Can you work these out from the model? Positions are in its coordinate system, mm. Face numbers are marked on the shaded views. A direction names the side the tool comes from. Round coordinates to 2 decimals unless told otherwise and drop trailing zeros. Write each loop counter-clockwise with the first axis right and the second up, starting at its lowest first coordinate (ties: lowest second). Pieces come first, ordered by that corner, then holes. Notation, with made-up numbers: M 24,52.5 L 69,52.5 A12 cw 69,58.5 Z; hole C 67,81 d4. An arc over 180 degrees is marked long. Use one line per item in the form item = value. Start each with the question number.
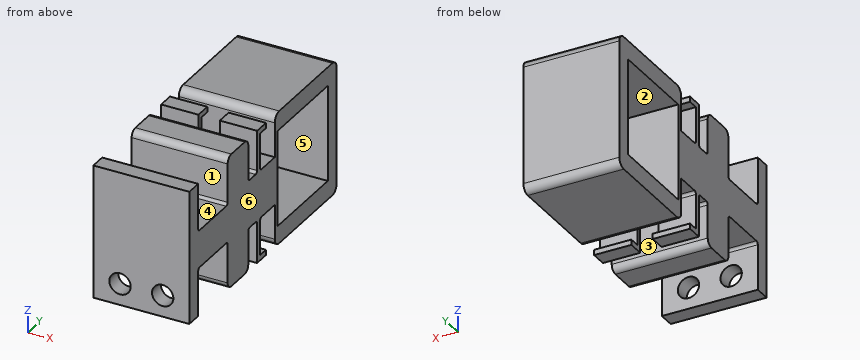
Autodesk Fusion 360 part; units mm, degrees
sketch "Sketch1" plane through (0, 0, 0) normal (1, 0, 0) x (0, 0, -1)
  line L0 (0, 0) -> (-18, 0)
  line L1 (-18, 0) -> (-18, 17)
  line L2 (-18, 17) -> (0, 17)
  line L3 (0, 17) -> (0, 0)
  line L4 (-21.5, 20) -> (3.5, 20)
  line L5 (3.5, 20) -> (3.5, -30)
  line L6 (3.5, -30) -> (-21.5, -30)
  line L7 (-21.5, -30) -> (-21.5, 20)
  dimension "d1" = 18
  dimension "d2" = 17
  dimension "d3" = 25
  dimension "d4" = 50
  dimension "d66" = 3.5
extrude "Extrude1" add sketch "Sketch1" against normal blind 18
fillet "Fillet1" radius 1.5 2 edges at (-9, 20, -3.5) (-9, 20, 21.5)
sketch "Sketch2" plane through (0, 0, 0) normal (1, 0, 0) x (0, 0, -1)
  line L0 (-18, 17) -> (0, 17)
  line L1 (0, 17) -> (0, 0)
  line L2 (0, 0) -> (-18, 0)
  line L3 (-18, 0) -> (-18, 17)
  arc A0 (-20, 20) -> (-21.5, 18.5) centre (-20, 18.5) ccw
  line L4 (-21.5, 18.5) -> (-21.5, -30)
  line L5 (-21.5, -30) -> (3.5, -30)
  line L6 (3.5, -30) -> (3.5, 18.5)
  arc A1 (3.5, 18.5) -> (2, 20) centre (2, 18.5) ccw
  line L7 (2, 20) -> (-20, 20)
  line L8 (-21.5, -3.9907) -> (-20.5, -3.9907)
  line L9 (-20.5, -3.9907) -> (-20.5, -6)
  line L10 (-20.5, -6) -> (-13.5, -6)
  line L11 (-13.5, -6) -> (-13.5, -0.9907)
  line L12 (-13.5, -0.9907) -> (-21.5, -0.9907)
  line L13 (3.5, -1) -> (-4.5, -1)
  line L14 (-4.5, -1) -> (-4.5, -6)
  line L15 (-4.5, -6) -> (2.5, -6)
  line L16 (2.5, -6) -> (2.5, -4)
  line L17 (2.5, -4) -> (3.5, -4)
  dimension "d9" = 7
  dimension "d10" = 8
  dimension "d12" = 5.0093
  dimension "d13" = 1
  dimension "d14" = 3
  dimension "d15" = 3
  dimension "d16" = 5
  dimension "d17" = 1
extrude "Extrude2" cut sketch "Sketch2" against normal blind 43 contours L4 L8 L9 L10 L11 L12 | L6 L13 L14 L15 L16 L17
sketch "Sketch3" plane through (0, 0, 21.5) normal (0, 0, 1) x (1, 0, 0)
  line L0 (0, -3.9907) -> (-18, -3.9907)
  line L1 (-18, -3.9907) -> (-18, -30)
  line L2 (-18, -30) -> (0, -30)
  line L3 (0, -30) -> (0, -3.9907)
  line L4 (0, -3.9907) -> (-7, -3.9907)
  line L5 (-7, -3.9907) -> (-7, -5.9907)
  line L6 (-7, -5.9907) -> (0, -5.9907)
  line L7 (0, -5.9907) -> (0, -3.9907)
  line L8 (-18, -3.9907) -> (-11, -3.9907)
  line L9 (-11, -3.9907) -> (-11, -5.9907)
  line L10 (-11, -5.9907) -> (-18, -5.9907)
  line L11 (-18, -5.9907) -> (-18, -3.9907)
  line L12 (-11, -3.9907) -> (-7, -3.9907)
  line L13 (-7, -3.9907) -> (-7, -5.9907)
  line L14 (-7, -5.9907) -> (-11, -5.9907)
  line L15 (-11, -5.9907) -> (-11, -3.9907)
  dimension "d21" = 7
  dimension "d22" = 2
  dimension "d23" = 7
  dimension "d24" = 2
extrude "Extrude3" cut sketch "Sketch3" against normal blind 8 contours L0 L5 L9 L12 L13 L14 L15
sketch "Sketch4" plane through (0, 0, -3.5) normal (0, 0, -1) x (-1, 0, 0)
  line L0 (18, -4) -> (0, -4)
  line L1 (0, -4) -> (0, -30)
  line L2 (0, -30) -> (18, -30)
  line L3 (18, -30) -> (18, -4)
  line L4 (0, -4) -> (7, -4)
  line L5 (7, -4) -> (7, -6)
  line L6 (7, -6) -> (0, -6)
  line L7 (0, -6) -> (0, -4)
  line L8 (18, -4) -> (11, -4)
  line L9 (11, -4) -> (11, -6)
  line L10 (11, -6) -> (18, -6)
  line L11 (18, -6) -> (18, -4)
  line L12 (7, -4) -> (11, -4)
  line L13 (11, -4) -> (11, -6)
  line L14 (11, -6) -> (7, -6)
  line L15 (7, -6) -> (7, -4)
  dimension "d27" = 7
  dimension "d28" = 2
  dimension "d29" = 7
  dimension "d30" = 2
extrude "Extrude4" cut sketch "Sketch4" against normal blind 8 contours L0 L5 L9 L12 L13 L14 L15
sketch "Sketch5" plane through (0, 0, -3.5) normal (0, 0, -1) x (-1, 0, 0)
  line L0 (7, -6) -> (7, -4)
  line L1 (7, -4) -> (0, -4)
  line L2 (0, -4) -> (0, -30)
  line L3 (0, -30) -> (18, -30)
  line L4 (18, -30) -> (18, -4)
  line L5 (18, -4) -> (11, -4)
  line L6 (11, -4) -> (11, -6)
  line L7 (11, -6) -> (7, -6)
  line L8 (7, -4) -> (11, -4)
  line L9 (11, -4) -> (11, -10)
  line L10 (11, -10) -> (7, -10)
  line L11 (7, -10) -> (7, -4)
  line L12 (11, -10) -> (18, -10)
  line L13 (18, -10) -> (18, -7)
  line L14 (18, -7) -> (11, -7)
  line L15 (11, -7) -> (11, -10)
  line L16 (7, -10) -> (0, -10)
  line L17 (0, -10) -> (0, -7)
  line L18 (0, -7) -> (7, -7)
  line L19 (7, -7) -> (7, -10)
  dimension "d33" = 3
extrude "Extrude5" cut sketch "Sketch5" against normal blind 8 contours L0 L6 L7 L8 L9 L11 | L7 L9 L10 L11 L15 L19 | L2 L11 L16 L17 L18 L19 | L4 L9 L12 L13 L14 L15
sketch "Sketch6" plane through (0, 0, 21.5) normal (0, 0, 1) x (1, 0, 0)
  line L0 (-11, -5.9907) -> (-11, -3.9907)
  line L1 (-11, -3.9907) -> (-18, -3.9907)
  line L2 (-18, -3.9907) -> (-18, -30)
  line L3 (-18, -30) -> (0, -30)
  line L4 (0, -30) -> (0, -3.9907)
  line L5 (0, -3.9907) -> (-7, -3.9907)
  line L6 (-7, -3.9907) -> (-7, -5.9907)
  line L7 (-7, -5.9907) -> (-11, -5.9907)
  line L8 (-11, -5.9907) -> (-7, -5.9907)
  line L9 (-7, -5.9907) -> (-7, -9.9907)
  line L10 (-7, -9.9907) -> (-11, -9.9907)
  line L11 (-11, -9.9907) -> (-11, -5.9907)
  line L12 (-7, -9.9907) -> (0, -9.9907)
  line L13 (0, -9.9907) -> (0, -6.9907)
  line L14 (0, -6.9907) -> (-7, -6.9907)
  line L15 (-7, -6.9907) -> (-7, -9.9907)
  line L16 (-11, -9.9907) -> (-18, -9.9907)
  line L17 (-18, -9.9907) -> (-18, -6.9907)
  line L18 (-18, -6.9907) -> (-11, -6.9907)
  line L19 (-11, -6.9907) -> (-11, -9.9907)
  dimension "d36" = 4
  dimension "d37" = 3
  dimension "d38" = 3
  dimension "d39" = 7
extrude "Extrude6" cut sketch "Sketch6" against normal blind 8 contours L7 L8 L9 L10 L11 L15 L19 | L2 L11 L16 L17 L18 L19 | L4 L9 L12 L13 L14 L15
sketch "Sketch7" plane through (0, -30, 0) normal (0, -1, 0) x (1, 0, 0)
  line L0 (0, -3.5) -> (0, 21.5)
  line L1 (0, 21.5) -> (-18, 21.5)
  line L2 (-18, 21.5) -> (-18, -3.5)
  line L3 (-18, -3.5) -> (0, -3.5)
sketch "Sketch8" plane through (0, 0, 0) normal (1, 0, 0) x (0, 0, -1)
  line L0 (-13.5, -9.9907) -> (-21.5, -9.9907)
  line L1 (-21.5, -9.9907) -> (-21.5, -30)
  line L2 (-21.5, -30) -> (3.5, -30)
  line L3 (3.5, -30) -> (3.5, -10)
  line L4 (3.5, -10) -> (-4.5, -10)
  line L5 (-4.5, -10) -> (-4.5, -7)
  line L6 (-4.5, -7) -> (3.5, -7)
  line L7 (3.5, -7) -> (3.5, -4)
  line L8 (3.5, -4) -> (2.5, -4)
  line L9 (2.5, -4) -> (2.5, -6)
  line L10 (2.5, -6) -> (-4.5, -6)
  line L11 (-4.5, -6) -> (-4.5, -1)
  line L12 (-4.5, -1) -> (3.5, -1)
  line L13 (3.5, -1) -> (3.5, 18.5)
  arc A0 (3.5, 18.5) -> (2, 20) centre (2, 18.5) ccw
  line L14 (2, 20) -> (-20, 20)
  arc A1 (-20, 20) -> (-21.5, 18.5) centre (-20, 18.5) ccw
  line L15 (-21.5, 18.5) -> (-21.5, -0.9907)
  line L16 (-21.5, -0.9907) -> (-13.5, -0.9907)
  line L17 (-13.5, -0.9907) -> (-13.5, -6)
  line L18 (-13.5, -6) -> (-20.5, -6)
  line L19 (-20.5, -6) -> (-20.5, -3.9907)
  line L20 (-20.5, -3.9907) -> (-21.5, -3.9907)
  line L21 (-21.5, -3.9907) -> (-21.5, -6.9907)
  line L22 (-21.5, -6.9907) -> (-13.5, -6.9907)
  line L23 (-13.5, -6.9907) -> (-13.5, -9.9907)
  line L24 (-18, 17) -> (0, 17)
  line L25 (0, 17) -> (0, 0)
  line L26 (0, 0) -> (-18, 0)
  line L27 (-18, 0) -> (-18, 17)
  line L28 (-21.5, -30) -> (3.5, -30)
  line L29 (3.5, -30) -> (3.5, -27)
  line L30 (3.5, -27) -> (-21.5, -27)
  line L31 (-21.5, -27) -> (-21.5, -30)
  line L32 (-21.5, -27) -> (-12.5, -27)
  line L33 (-12.5, -27) -> (-12.5, -23)
  line L34 (-12.5, -23) -> (-21.5, -23)
  line L35 (-21.5, -23) -> (-21.5, -27)
  line L36 (3.5, -27) -> (-5.5, -27)
  line L37 (-5.5, -27) -> (-5.5, -23)
  line L38 (-5.5, -23) -> (3.5, -23)
  line L39 (3.5, -23) -> (3.5, -27)
  dimension "d42" = 3
extrude "Extrude7" cut sketch "Sketch8" against normal blind 32 contours L1 L30 L32 L33 L34 L35 | L3 L30 L36 L37 L38 L39
fillet "Fillet2" radius 0.5 8 edges at (-14.5, -6, 13.5) (-3.5, -6, 13.5) (-3.5, -6.9907, 13.5) (-14.5, -6.9907, 13.5) (-3.5, -7, 4.5) (-3.5, -6, 4.5) (-14.5, -6, 4.5) (-14.5, -7, 4.5)
sketch "Sketch9" plane through (0, -30, 0) normal (0, -1, 0) x (1, 0, 0)
  line L0 (0, 20) -> (-18, 20)
  line L1 (-18, 20) -> (-18, -5)
  line L2 (-18, -5) -> (0, -5)
  line L3 (0, -5) -> (0, 20)
  line L4 (0, 20) -> (0, 7.5)
  line L5 (0, 7.5) -> (-18, 7.5)
  line L6 (-18, 7.5) -> (-13, 7.5)
  circle A0 centre (-13, 0.5) radius 2
  line L7 (-9, -5) -> (-9, 20)
  circle A1 centre (-5, 0.5) radius 2
  dimension "d50" = 4
  dimension "d63" = 4
  dimension "d64" = 4
  dimension "d65" = 4
extrude "Extrude8" cut sketch "Sketch9" against normal blind 5 contours A0 | A1
extrude "Extrude9" cut 2 faces at (-12, -23, 15.5) (-12, -23, -0.5) along direction (0, 1, 0) blind 6
fillet "Fillet3" radius 1.25 4 edges at (-9, -9.9907, 21.5) (-9, -17, 21.5) (-9, -10, -3.5) (-9, -17, -3.5)
fillet "Fillet4" radius 0.5 4 edges at (-9, -10, 4.5) (-9, -17, 5.5) (-9, -17, 12.5) (-9, -9.9907, 13.5)
fillet "Fillet5" radius 0.5 2 edges at (-9, -27, 12.5) (-9, -27, 5.5)
fillet "Fillet6" radius 1.5 2 edges at (-9, -1, -3.5) (-9, -0.9907, 21.5)
1. If we mould it in two halves opening along Z, with no side actions, what happens to the marked faces 4, 5 and 6? For each: pulls with the +Z half, pulls with the -Z half, needs draft (parallel to the pull), parting line crosses it, or undercut.
2. Please list where these lines run through material, in increasing order: line 1 along Y through (x, z) = (-7.25, -0.5); line 2 along Y through (x, z) = (-15.75, 15.25); line 3 along Y through (x, z) = (-4.5, -1.5).
3. Will these pins go through, and if not, where does the flat tip stop? pin 1 (2.5 mm diameter, centred on x = -5, z = 0.5, fed in from -Y); pin 2 (1.5 mm diameter, centred on y = -13.5, z = 13.5, fed in from +X).
4. If we section it at A-A (z = 0.5): State how many separate pieces and enclosed holes the cut face has, and give its area (3 significant figures).
5. If we section it at B-B (y = 9): List the corners of the cut face in (x, z) for me, and give its area (3 significant figures).
6. If we section it at C-C (y = -4.5): List the corners of the cut face in (x, z) for me, and give its area (3 significant figures).
7. Which directions (+Z, -Z, +X, -X, +Y, -Y) give clear straight access to the entire face, cutting with the end or side of a thin tool? Please do the marked faces 1, 2 and 3.
Model answer:
q1.face_4 = pulls with the +Z half
q1.face_5 = undercut
q1.face_6 = needs draft
q2.line_1 = -30 to -27, -17 to -10, -1 to 20
q2.line_2 = -30 to -27, -17 to -9.99, -6.99 to -6, -0.99 to 0, 17 to 20
q2.line_3 = -30 to -27, -17 to -10, -7 to -6, -1 to 20
q3.pin_1 = -17
q3.pin_2 = 0
q4.separate_pieces = 8
q4.enclosed_holes = 0
q4.area = 242 mm2
q5.outline = M -18,-3.5 L 0,-3.5 L 0,0 L -18,0 Z; M -18,18 L 0,18 L 0,21.5 L -18,21.5 Z
q5.area = 126 mm2
q6.outline = M -18,-3.5 L -11,-3.5 L -11,-2.5 L -18,-2.5 Z; M -18,4.5 L 0,4.5 L 0,13.5 L -18,13.5 Z; M -18,20.5 L -11,20.5 L -11,21.5 L -18,21.5 Z; M -7,-3.5 L 0,-3.5 L 0,-2.5 L -7,-2.5 Z; M -7,20.5 L 0,20.5 L 0,21.5 L -7,21.5 Z
q6.area = 190 mm2
q7.face_1 = +Z, +X, -X
q7.face_2 = +X, -X
q7.face_3 = -Z, +X, -X
